```python
from build123d import *

# Parameters (mm, degrees)
BOSS_EXTRU_1_DEPTH              = 179.2
BOSS_EXTRU_1_DEPTH_BACK         = 2
ESQUISSE1_W                     = 10
ESQUISSE1_H                     = 10
ESQUISSE2_W                     = 2
ESQUISSE2_H                     = 10
ESQUISSE2_W_2                   = 5
ENL_V_MAT_EXTRU_1_DEPTH         = 180.548433577
TROU_TARAUD_M3X0_51_D           = 2.5
TROU_TARAUD_M3X0_51_CSINK_D     = 3.05
TROU_TARAUD_M3X0_51_CSINK_ANGLE = 90
TROU_TARAUD_M3X0_52_D           = 2.5
TROU_TARAUD_M3X0_52_DEPTH       = 8.5


with BuildPart() as part:
    # Esquisse1 → Boss.-Extru.1 (new, two sides: drawn at the far end of the back side and taken through both)
    with BuildSketch(Plane.XY.offset(-BOSS_EXTRU_1_DEPTH_BACK)):
        Rectangle(ESQUISSE1_W, ESQUISSE1_H)
    extrude(amount=BOSS_EXTRU_1_DEPTH + BOSS_EXTRU_1_DEPTH_BACK)

    # Esquisse2 → Enlèv. mat.-Extru.1 (cut, through all)
    with BuildSketch(Plane(origin=(0, 5, 0), x_dir=(1, 0, 0), z_dir=(0, 1, 0))):
        with Locations((4, -122.2)):
            Rectangle(ESQUISSE2_W, ESQUISSE2_H)
        with Locations((4, -21.2)):
            Rectangle(ESQUISSE2_W, ESQUISSE2_H)
        with Locations((2.5, -47.4)):
            Rectangle(ESQUISSE2_W_2, ESQUISSE2_H)
    extrude(amount=-ENL_V_MAT_EXTRU_1_DEPTH, mode=Mode.SUBTRACT)

    # Trou taraudé M3x0.51 (through all)
    with Locations(Plane(origin=(0, 5, 0), x_dir=(1, 0, 0), z_dir=(0, 1, 0))):
        with Locations((0, -10)):
            CounterSinkHole(TROU_TARAUD_M3X0_51_D / 2, TROU_TARAUD_M3X0_51_CSINK_D / 2, counter_sink_angle=TROU_TARAUD_M3X0_51_CSINK_ANGLE)

    # Trou taraudé M3x0.52
    with Locations(Plane.XY.offset(179.2)):
        with Locations((0, 0)):
            Hole(TROU_TARAUD_M3X0_52_D / 2, depth=TROU_TARAUD_M3X0_52_DEPTH)


solid = part.part
```
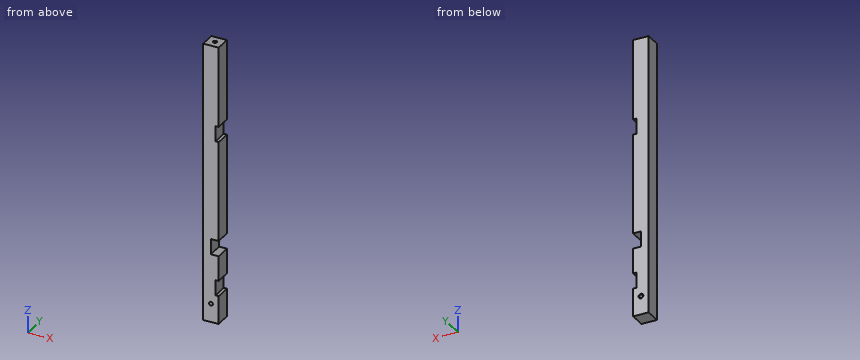
Read the model definition and answer for the solid it produces. Units are mm, in the model's axes. Give positions to 0.01 mm unless a question says otherwise; leave off trailing zeros. Write each loop counter-clockwise with the first axis right and the second up, starting at its lowest first coordinate (ties: lowest second). Pieces come first, ordered by that corner, then holes. Notation, with made-up numbers: (5, -28) - (28, -28) arc R21 cw to (28, 5) - close; hole circle Ø1 at (13.5, 5.5). An arc over 180 degrees is marked (long way). Write item = value, one per line. Start each with the question number.
Item 1: Each of these flat-tipped pins is pushed along its axis until it touches: P1, Ø3, axis at x = 0, y = 0, coming from the +Z side; P2, Ø3, axis at y = 1, z = 49, coming from the +X side; P3, Ø3, axis at y = 0.5, z = 18.5, coming from the +X side. Where does it stop, or does it pass through?
Item 2: Find the intervals of material crossed by probe 1 along Z at (x, y) = (3.25, -1.25); probe 2 along Y at (x, z) = (0, 175.75); probe 3 along Z at (x, y) = (2.25, -1.75), in increasing order. Write a range as [from, to].
Item 3: Find section A-A (y = 3). Give the vertices of the cut face in (x, z).
Item 4: Find section B-B (z = 19.5). Give the vertices of the cut face in (x, y), then the cut area to 3 significant figures.
Response:
q1.P1 = 179.2
q1.P2 = 0
q1.P3 = 3
q2.probe_1 = [-2, 16.2], [26.2, 42.4], [52.4, 117.2], [127.2, 179.2]
q2.probe_2 = [-5, -1.25], [1.25, 5]
q2.probe_3 = [-2, 42.4], [52.4, 179.2]
q3.outline = (-5, -2) - (5, -2) - (5, 16.2) - (3, 16.2) - (3, 26.2) - (5, 26.2) - (5, 42.4) - (0, 42.4) - (0, 52.4) - (5, 52.4) - (5, 117.2) - (3, 117.2) - (3, 127.2) - (5, 127.2) - (5, 179.2) - (-5, 179.2) - close; hole circle Ø2.5 at (0, 10)
q4.outline = (-5, -5) - (3, -5) - (3, 5) - (-5, 5) - close
q4.area = 80.0 mm²
